Here's how the part is built. I have some questions about the finished solid (model axes, mm). Round coordinates to 2 decimals unless told otherwise and drop trailing zeros. Loops run counter-clockwise (first coordinate to the right, second up) from the corner with the lowest first, then second, coordinate; pieces in that order, holes last. Notation, with made-up numbers: M -31,38.25 L -6,38.25 A23 cw -6,52.25 Z; hole C 50.5,88 d2. An arc over 180 degrees is marked long. Answer as a JSON object with one key per item and string values.
from build123d import *

# Parameters (mm, degrees)
F1_DEPTH    = 1381.125
F2_R        = 1.5875
F3_T1_DEPTH = 2767.5102424874
F3_T3_DEPTH = 2765.8360222341


# Not quite as in the source:
# - a fillet or chamfer that OpenCascade refuses, or shapes differently, is made with other operations: its cross-section is extruded or revolved along the edge and cut away or added


with BuildPart() as f1:
    # F0 (on Front) → F1 (new body, symmetric)
    with BuildSketch(Plane.XZ):
        with BuildLine():
            Line((0, 16.6624), (0, 0))
            Line((0, 0), (41.275, 0))
            Line((41.275, 0), (41.275, 16.6624))
            ThreePointArc((41.275, 16.6624), (37.3126, 20.6248), (33.3502, 16.6624))
            Line((33.3502, 16.6624), (34.9377, 16.6624))
            ThreePointArc((34.9377, 16.6624), (37.3126, 19.0373), (39.6875, 16.6624))
            Line((39.6875, 16.6624), (39.6875, 1.5875))
            Line((39.6875, 1.5875), (1.5875, 1.5875))
            Line((1.5875, 1.5875), (1.5875, 16.6624))
            ThreePointArc((1.5875, 16.6624), (3.9624, 19.0373), (6.3373, 16.6624))
            Line((6.3373, 16.6624), (7.9248, 16.6624))
            ThreePointArc((7.9248, 16.6624), (3.9624, 20.6248), (0, 16.6624))
        make_face()
    extrude(amount=F1_DEPTH, both=True)

    # F2
    f2_edges = [f1.edges().sort_by_distance(p)[0] for p in [
        (41.275, 0, 0),
        (0, 0, 0),
        (39.6875, 0, 1.5875),
        (1.5875, 0, 1.5875),
    ]]
    fillet(f2_edges, radius=F2_R)

    # F3: fillet of radius 0.8255 on 4 edges, made by hand

    # F3_s2 → F3_t1 (cut)
    with BuildSketch(Plane.XZ.offset(-1383.7551212437)):
        with BuildLine():
            ThreePointArc((7.7851364071, 17.7051368421), (7.6447738654, 16.9868405041), (6.9887329889, 16.6624))
            Line((6.9887329889, 16.6624), (7.9248, 16.6624))
            ThreePointArc((7.9248, 16.6624), (7.889728895, 17.1884242487), (7.7851364071, 17.7051368421))
        make_face()
        with BuildLine():
            ThreePointArc((33.4898635929, 17.7051368421), (33.6302261346, 16.9868405041), (34.2862670111, 16.6624))
            Line((34.2862670111, 16.6624), (33.3502, 16.6624))
            ThreePointArc((33.3502, 16.6624), (33.385271105, 17.1884242487), (33.4898635929, 17.7051368421))
        make_face()
    extrude(amount=F3_T1_DEPTH, mode=Mode.SUBTRACT)

    # F3_s4 → F3_t3 (cut)
    with BuildSketch(Plane.XZ.offset(-1382.918011117)):
        with BuildLine():
            ThreePointArc((6.2569378236, 17.2749734127), (6.551672789, 16.8332164322), (7.0545044468, 16.6624))
            Line((7.0545044468, 16.6624), (6.3373, 16.6624))
            ThreePointArc((6.3373, 16.6624), (6.317123751, 16.9713110978), (6.2569378236, 17.2749734127))
        make_face()
        with BuildLine():
            ThreePointArc((34.2204955532, 16.6624), (34.723327211, 16.8332164322), (35.0180621764, 17.2749734127))
            ThreePointArc((35.0180621764, 17.2749734127), (34.957876249, 16.9713110978), (34.9377, 16.6624))
            Line((34.9377, 16.6624), (34.2204955532, 16.6624))
        make_face()
    extrude(amount=F3_T3_DEPTH, mode=Mode.SUBTRACT)


solid = f1.part
Item 1: I want a section at A-A on z = 12. List the corners of the cut face in (x, y) for me (1 decimal).
Solution:
{"outline": "M 0,-1381.1 L 1.6,-1381.1 L 1.6,1381.1 L 0,1381.1 Z; M 39.7,-1381.1 L 41.3,-1381.1 L 41.3,1381.1 L 39.7,1381.1 Z"}
Item 2: I want a section at B-B on y = -725. List the corners of the cut face in (x, z) for me (1 decimal).
Solution:
{"outline": "M 0,1.6 A1.6 ccw 1.6,0 L 39.7,0 A1.6 ccw 41.3,1.6 L 41.3,16.7 A4 ccw 33.5,17.7 A0.8 ccw 34.3,16.7 A0.8 ccw 35,17.3 A2.4 cw 39.7,16.7 L 39.7,3.2 A1.6 cw 38.1,1.6 L 3.2,1.6 A1.6 cw 1.6,3.2 L 1.6,16.7 A2.4 cw 6.3,17.3 A0.8 ccw 7,16.7 A0.8 ccw 7.8,17.7 A4 ccw 0,16.7 Z"}
Item 3: I want a section at C-C on x = 23. List the corners of the cut face in (y, z) for me (1 decimal).
Solution:
{"outline": "M -1381.1,0 L 1381.1,0 L 1381.1,1.6 L -1381.1,1.6 Z"}
Item 4: For P1, Ø1, axis at x = 16.5, y = 712.5, coming from the +Z side, with a flat end and sliding along its axis, tell me the tip position at first contact or that it passes through.
Solution:
{"P1": "stops at z = 1.59"}
Item 5: If I drill on L1, parallel to X at y = -696, z = 17.5; L2, parallel to X at y = 134.5, z = 14.5 (1 decimal); L3, parallel to Z at x = 37.5, y = 800, over which ranges is the centre line in solid material (lowest first)? Write a range as from..to.
Solution:
{"L1": "x = 0.09..1.74, 6.18..7.81, 33.46..35.09, 39.53..41.19", "L2": "x = 0..1.6, 39.7..41.3", "L3": "z = 0..1.59, 19.03..20.62"}
